Check sheet for the drawn part. Datum: minimum x, y, z corner. Units: mm. Coordinates: 2 decimals unless noted, no trailing zeros. Order: outer loops, then holes, each group sorted by start corner. A loop starts at its lowest first (then second) coordinate and runs counter-clockwise, first axis right, second up. Notation, with made-up numbers: (-38, 77.5) - (-1, 77.5) arc R16 ccw to (-1, 100.5) - close; hole circle Ø5 at (37.5, 12.5). An arc over 180 degrees is marked (long way). Answer as CSV lines item,"result". Start each with the question number.
1. Material ranges on L1, parallel to X at y = 6, z = 1.6 (3 decimals); L2, parallel to Y at x = 108, z = 1.4; L3, parallel to X at y = 19, z = 0.85 (3 decimals), recorded low to high. Write a range as [from, to].
2. Section check A-A (y = 66). Record the cut outline in (x, z) (3 decimals).
3. Section check B-B (x = 120.5). Record the cut outline in (y, z) (3 decimals), and give its area (3 significant figures).
4. Go/stop test with flat-tipped pins: pin 1 (1 mm diameter, centred on y = 10, z = 1, fed in from -X) (3 decimals); pin 2 (1.6 mm diameter, centred on y = 36.5, z = 1.5, fed in from +X) (3 decimals); pin 3 (1.6 mm diameter, centred on y = 2.5, z = 2, fed in from -X) (3 decimals). Record where each tip stops, or that it passes through.
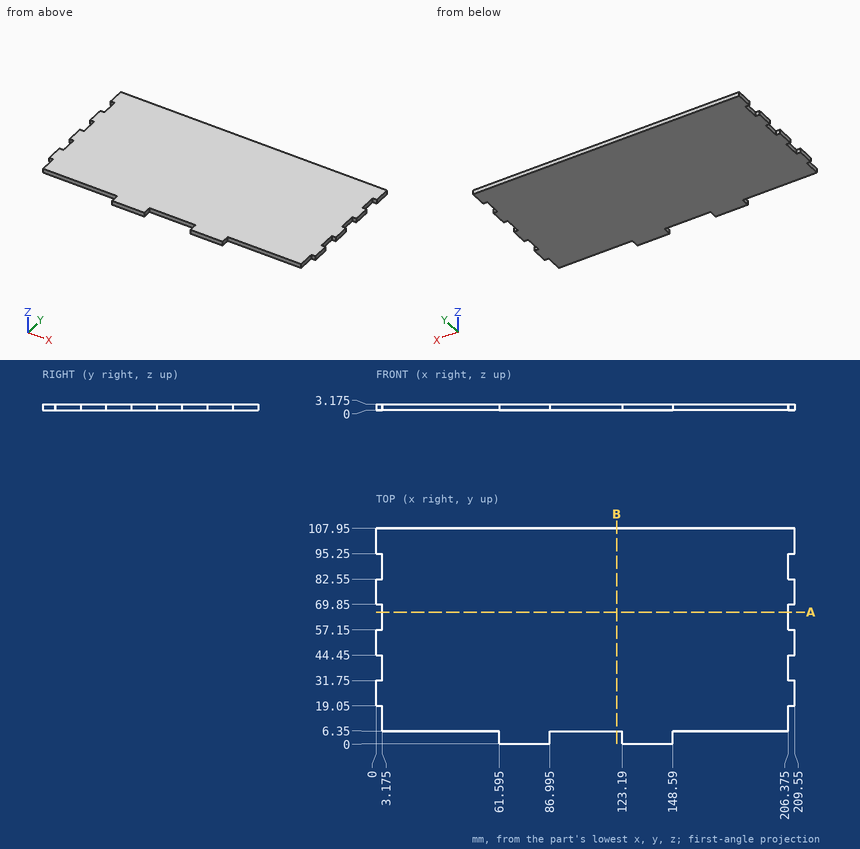
Evaluation:
1,L1,"x = [61.595, 86.995], [123.19, 148.59]"
1,L2,"y = [6.35, 107.95]"
1,L3,"x = [3.175, 206.375]"
2,outline,"(3.175, 0) - (206.375, 0) - (206.375, 3.175) - (3.175, 3.175) - close"
3,outline,"(6.35, 0) - (107.95, 0) - (107.95, 3.175) - (6.35, 3.175) - close"
3,area,"323 mm²"
4,pin 1,"stops at x = 3.175"
4,pin 2,"stops at x = 206.375"
4,pin 3,"stops at x = 61.595"
